Could you check a few things on this drawing? It's one solid part, dimensions in mm from its lowest x, y, z. Give positions to 0.01 mm unless a question says otherwise; leave off trailing zeros. Loops run counter-clockwise (first coordinate to the right, second up) from the corner with the lowest first, then second, coordinate; pieces in that order, holes last.
1. Imagine slicing it at D-D (y = 4.65). List the corners of the cut face in (x, z) for me, plus the area to 3 significant figures.
2. Imagine slicing it at C-C (z = 19). List the corners of the cut face in (x, y) for me.
3. Imagine slicing it at A-A (z = 32.5). List the corners of the cut face in (x, y) for me.
4. Imagine slicing it at B-B (y = 0.7). List the corners of the cut face in (x, z) for me (3 decimals).
5. I need wall thicknesses on line 1 along Y through (x, z) = (2.5, 29.5); line 2 along Y through (x, z) = (1.9, 29.5); line 3 along X through (y, z) = (2.65, 18). Which ranges of each line are inside material? Lowest first, please.
6. For P1, Ø1.5, axis at x = 4, z = 16.5, coming from the +Y side (3 decimals); P2, Ø1, axis at x = 3.5, z = 19.5, coming from the -Y side; P3, Ø1.5, axis at y = 1, z = 22.5, coming from the -X side (3 decimals), each with a flat end and sliding along its axis, tell me the tip position at first contact or that it passes through.
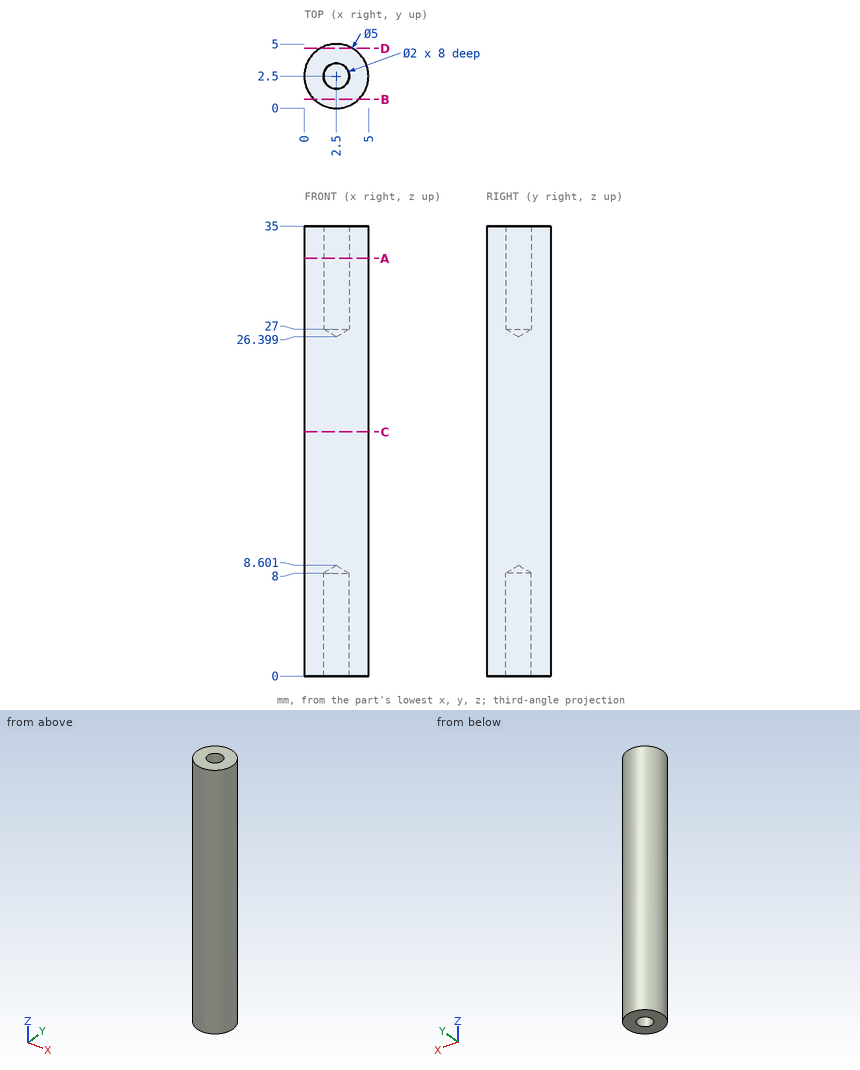
Derived:
1. outline: (1.22, 0) - (3.78, 0) - (3.78, 35) - (1.22, 35) - close
1. area: 89.3 mm2
2. outline: circle Ø5 at (2.5, 2.5)
3. outline: circle Ø5 at (2.5, 2.5); hole circle Ø2 at (2.5, 2.5)
4. outline: (0.765, 0) - (4.235, 0) - (4.235, 35) - (0.765, 35) - close
5. line 1: y = 0 to 1.5, 3.5 to 5
5. line 2: y = 0.07 to 1.7, 3.3 to 4.93
5. line 3: x = 0 to 5
6. P1: stops at y = 4.885
6. P2: stops at y = 0.05
6. P3: stops at x = 0.115
